```python
from build123d import *

# Parameters (mm, degrees)
PAD_DEPTH    = 5
FILLET_R     = 1
FILLET001_R  = 1
CHAMFER_SIZE = 4
FILLET002_R  = 3
FILLET003_R  = 1


with BuildPart() as part:
    # Sketch (on CopyPart__Feature) → Pad (new body)
    with BuildSketch(Plane(origin=(211.803644, 488.825915, 357.796851), x_dir=(-1, 0, 0), z_dir=(0, 0, 1))):
        Polygon((3.2, 28.8), (-0.4, 28.8), (-0.4, -0.75), (7.8, -0.75), (7.8, 3.7), (17.92547, 3.7), (17.92547, -2.5), (7.8, -2.5), (-2.4, -2.5), (-2.4, 35.8), (11.3, 35.8), (11.3, 28.8), (6.3, 28.8), (6.3, 33.8), (3.2, 33.8), align=None)
    extrude(amount=PAD_DEPTH)

    # Fillet
    fillet_edges = [part.edges().sort_by_distance(p)[0] for p in [
        (204.003644, 489.575915, 360.296851),
        (212.203644, 489.575915, 360.296851),
        (212.203644, 460.025915, 360.296851),
        (205.503644, 460.025915, 360.296851),
    ]]
    fillet(fillet_edges, radius=FILLET_R)

    # Fillet001
    fillet001_edges = [part.edges().sort_by_distance(p)[0] for p in [
        (208.603644, 460.025915, 360.296851),
        (208.603644, 455.025915, 360.296851),
    ]]
    fillet(fillet001_edges, radius=FILLET001_R)

    # Chamfer
    chamfer_edges = [part.edges().sort_by_distance(p)[0] for p in [
        (193.878174, 485.125915, 360.296851),
    ]]
    chamfer(chamfer_edges, length=CHAMFER_SIZE)

    # Fillet002
    fillet002_edges = [part.edges().sort_by_distance(p)[0] for p in [
        (197.878174, 485.125915, 360.296851),
    ]]
    fillet(fillet002_edges, radius=FILLET002_R)

    # Fillet003
    fillet003_edges = [part.edges().sort_by_distance(p)[0] for p in [
        (204.003644, 485.125915, 360.296851),
    ]]
    fillet(fillet003_edges, radius=FILLET003_R)


solid = part.part
```
Could you check a few things on this model? Use its own coordinates, in mm. A direction names the side the tool comes from. Round coordinates to 2 decimals unless told otherwise and drop trailing zeros. Order: outer loops, then holes, each group sorted by start corner. A loop starts at its lowest first (then second) coordinate and runs counter-clockwise, first axis right, second up. Notation, with made-up numbers: (0, 7.5) -> (23, 7.5) arc R15 ccw to (23, 31.5) -> close; hole circle Ø2 at (56, -3.5). An arc over 180 degrees is marked (long way). One line per question, with ' | ' between items.
Q1. Which directions (+Z, -Z, +X, -X, +Y, -Y) give clear straight access to the entire face, cutting with the end or side of a thin tool? Please do faces 1 (the face through (208.32, 455.33, 360.33)), 2 (the face through (202, 460.026, 360)), 3 (the face through (213, 471, 357.797)).
Computed values:
face 1: +Z, -Z | face 2: +Z, -Z, -X | face 3: -Z, +X, -X, +Y, -Y
Q2. If we section it at A-A on y = 457: Write out the boundary of the cut face in (x, z).
Computed values:
outline: (200.5, 357.8) -> (205.5, 357.8) -> (205.5, 362.8) -> (200.5, 362.8) -> close; (208.6, 357.8) -> (214.2, 357.8) -> (214.2, 362.8) -> (208.6, 362.8) -> close
Q3. If we section it at D-D on y = 463: Write out the boundary of the cut face in (x, z), plus the area to 4 significant figures.
Computed values:
outline: (212.2, 357.8) -> (214.2, 357.8) -> (214.2, 362.8) -> (212.2, 362.8) -> close | area: 10.00 mm²
Q4. We'd pull the mould along Y, two halves only. Please class faces 4 (the face through (200.504, 456, 360)), 5 (the face through (201, 485.126, 360)), 6 (the face through (212.204, 475, 360)), 7 (the face through (197.988, 485.348, 360.332)): released by +Y, released by -Y, zero draft, split by the parting line, or undercut.
Computed values:
face 4: zero draft | face 5: undercut | face 6: undercut | face 7: released by -Y
Q5. If we section it at C-C on z = 359.25: Write out the boundary of the cut face in (x, y), plus the area to 3 significant figures.
Computed values:
outline: (193.88, 489.13) -> (197, 486) arc R3 ccw to (199.12, 485.13) -> (203, 485.13) arc R1 ccw to (204, 486.13) -> (204, 488.58) arc R1 cw to (205, 489.58) -> (211.2, 489.58) arc R1 cw to (212.2, 488.58) -> (212.2, 461.03) arc R1 cw to (211.2, 460.03) -> (209.6, 460.03) arc R1 ccw to (208.6, 459.03) -> (208.6, 456.03) arc R1 cw to (207.6, 455.03) -> (205.5, 455.03) -> (205.5, 459.03) arc R1 ccw to (204.5, 460.03) -> (200.5, 460.03) -> (200.5, 453.03) -> (214.2, 453.03) -> (214.2, 491.33) -> (193.88, 491.33) -> close | area: 212 mm²
Q6. If I drill on line 1 (Y direction, x = 206.5, z = 360.2); line 2 (Y direction, x = 203, z = 359.5); line 3 (X direction, y = 458.5, z = 360.65), over which ranges is the centre line in solid material (lowest first)? Write a range as from..to.
Computed values:
line 1: 453.03..455.03, 489.58..491.33 | line 2: 453.03..460.03, 485.13..491.33 | line 3: 200.5..205.5, 208.6..214.2
Q7. I'm going to push flat-ended pins straight in: pin 1 (1.5 mm diameter, centred on y = 480, z = 359, fed in from -X); pin 2 (0.9 mm diameter, centred on y = 457, z = 359, fed in from -X); pin 3 (2 mm diameter, centred on y = 485, z = 359, fed in from -X); pin 4 (1 mm diameter, centred on x = 198, y = 485, fed in from -Z). Where does each tip first touch, or does it pass through?
Computed values:
pin 1: x = 212.2 | pin 2: x = 200.5 | pin 3: x = 197 | pin 4: z = 357.8
Q8. If we section it at B-B on x = 201.5: Write out the boundary of the cut face in (y, z).
Computed values:
outline: (453.03, 357.8) -> (460.03, 357.8) -> (460.03, 362.8) -> (453.03, 362.8) -> close; (485.13, 357.8) -> (491.33, 357.8) -> (491.33, 362.8) -> (485.13, 362.8) -> close
